```python
from build123d import *

# Parameters (mm, degrees)
BOSS_EXTRUDE1_DEPTH = 34
SKETCH2_R           = 1.5
CUT_EXTRUDE1_DEPTH  = 49.887626246
SKETCH3_R           = 1.25
SKETCH3_R_2         = 0.75
CUT_EXTRUDE2_DEPTH  = 48.759815745


with BuildPart() as part:
    # Sketch1 → Boss-Extrude1 (new body)
    with BuildSketch(Plane(origin=(0, 0, 0), x_dir=(0, 0, -1), z_dir=(1, 0, 0))):
        Polygon((0, 0), (6, 0), (6, 35), (3, 35), (3, 2), (0, 2), align=None)
    extrude(amount=BOSS_EXTRUDE1_DEPTH)

    # Sketch2 → Cut-Extrude1 (cut, through all)
    with BuildSketch(Plane.XY.offset(-3)):
        with Locations((29.2, 31.2)):
            Circle(SKETCH2_R)
        with Locations((4.8, 31.2)):
            Circle(SKETCH2_R)
        with Locations((4.8, 6.8)):
            Circle(SKETCH2_R)
        with Locations((29.2, 6.8)):
            Circle(SKETCH2_R)
    extrude(amount=-CUT_EXTRUDE1_DEPTH, mode=Mode.SUBTRACT)

    # Sketch3 → Cut-Extrude2 (cut, through all)
    with BuildSketch(Plane(origin=(0, 2, 0), x_dir=(1, 0, 0), z_dir=(0, 1, 0))):
        with Locations(Location((17, 1.5, 0), (0, 0, 270))):
            Circle(SKETCH3_R)
        with Locations(Location((22, 1.5, 0), (0, 0, 270))):
            Circle(SKETCH3_R_2)
        with Locations(Location((25, 1.5, 0), (0, 0, 270))):
            Circle(SKETCH3_R_2)
        with Locations(Location((12, 1.5, 0), (0, 0, 270))):
            Circle(SKETCH3_R_2)
        with Locations(Location((9, 1.5, 0), (0, 0, 270))):
            Circle(SKETCH3_R_2)
    extrude(amount=-CUT_EXTRUDE2_DEPTH, mode=Mode.SUBTRACT)


solid = part.part
```
Geometry check sheet. Reference: the model listing, model coordinates, mm. A direction names the side the tool comes from. Give positions to 0.01 mm unless a question says otherwise; leave off trailing zeros. Order: outer loops, then holes, each group sorted by start corner. A loop starts at its lowest first (then second) coordinate and runs counter-clockwise, first axis right, second up. Notation, with made-up numbers: (7.5, 18) - (24.5, 18) arc R25 cw to (24.5, 36) - close; hole circle Ø3 at (4, -2). An arc over 180 degrees is marked (long way). Answer in a Markdown table with one row per item. Add a question column.
Q1. Tool access check on faces 1 (the flat face through (17, 19, -3)), 2 (the flat face through (17, 35, -5)). Record the directions out of +Z, -Z, +X, -X, +Y, -Y that give a thin tool (end or side, any length) a straight path to the whole face; none if there is none.
Q2. Gauge pin test, flat ends, axial feed: pin 1 (1.8 mm diameter, centred on x = 29.2, y = 31.2, fed in from +Z); pin 2 (3 mm diameter, centred on x = 23.5, y = 7, fed in from +Z); pin 3 (1.5 mm diameter, centred on x = 19, z = -2, fed in from +Y). Record the tip position at first contact, or that the pin passes through.
Q3. Material ranges on probe 1 along Y at (x, z) = (4.8, -4.45); probe 2 along X at (y, z) = (0.7, -1.5); probe 3 along Y at (x, z) = (3.5, -3.9), recorded low to high. Write a range as from..to.
Q4. Cross-section at A-A, the plane x = 4.8. Enter the section's corners in (y, z), then the cut area to 3 significant figures.
Q5. Cross-section at D-D, the plane z = -4. Enter the section's corners in (x, y).
Q6. Cross-section at C-C, the plane x = 9. Enter the section's corners in (y, z).
Q7. Cross-section at B-B, the plane y = 6.8. Enter the section's corners in (x, z).
Q8. Mould release check, pull along X, two halves, no side actions. Record for faces 3 (the flat face through (0, 18, -4)), 4 (the flat face through (21, 2, -2)), 5 (the cylindrical face through (9.632, 1.014, -1.097)): pulls with the +X half, pulls with the -X half, needs draft (parallel to the pull), parting line crosses it, or undercut.
Check values:
| question | item | result |
|---|---|---|
| 1 | face 1 | +Z, +X, -X, +Y |
| 1 | face 2 | +Z, -Z, +X, -X, +Y |
| 2 | pin 1 | passes through |
| 2 | pin 2 | stops at z = -3 |
| 2 | pin 3 | stops at y = 2 |
| 3 | probe 1 | y = 0..5.3, 8.3..29.7, 32.7..35 |
| 3 | probe 2 | x = 0..8.25, 9.75..11.25, 12.75..15.75, 18.25..21.25, 22.75..24.25, 25.75..34 |
| 3 | probe 3 | y = 0..6.05, 7.55..30.45, 31.95..35 |
| 4 | outline | (0, -6) - (5.3, -6) - (5.3, -3) - (2, -3) - (2, 0) - (0, 0) - close; (8.3, -6) - (29.7, -6) - (29.7, -3) - (8.3, -3) - close; (32.7, -6) - (35, -6) - (35, -3) - (32.7, -3) - close |
| 4 | area | 93.0 mm^2 |
| 5 | outline | (0, 0) - (34, 0) - (34, 35) - (0, 35) - close; hole circle Ø3 at (4.8, 6.8); hole circle Ø3 at (4.8, 31.2); hole circle Ø3 at (29.2, 6.8); hole circle Ø3 at (29.2, 31.2) |
| 6 | outline | (0, -6) - (35, -6) - (35, -3) - (2, -3) - (2, -2.25) - (0, -2.25) - close; (0, -0.75) - (2, -0.75) - (2, 0) - (0, 0) - close |
| 7 | outline | (0, -6) - (3.3, -6) - (3.3, -3) - (0, -3) - close; (6.3, -6) - (27.7, -6) - (27.7, -3) - (6.3, -3) - close; (30.7, -6) - (34, -6) - (34, -3) - (30.7, -3) - close |
| 8 | face 3 | pulls with the -X half |
| 8 | face 4 | needs draft |
| 8 | face 5 | undercut |
